Check sheet for the drawn part. Datum: minimum x, y, z corner. Units: mm. A direction names the side the tool comes from. Give positions to 0.01 mm unless a question says otherwise; leave off trailing zeros. Write each loop counter-clockwise with the first axis right and the second up, starting at its lowest first coordinate (ties: lowest second). Pieces come first, ordered by that corner, then holes. Notation, with made-up numbers: (22, 60.25) -> (66, 60.25) arc R24 ccw to (66, 86.25) -> close; hole circle Ø3 at (-30, -9). An arc over 180 degrees is marked (long way). Use CSV: the item, a comma, the result in double quotes. Start each with the question number.
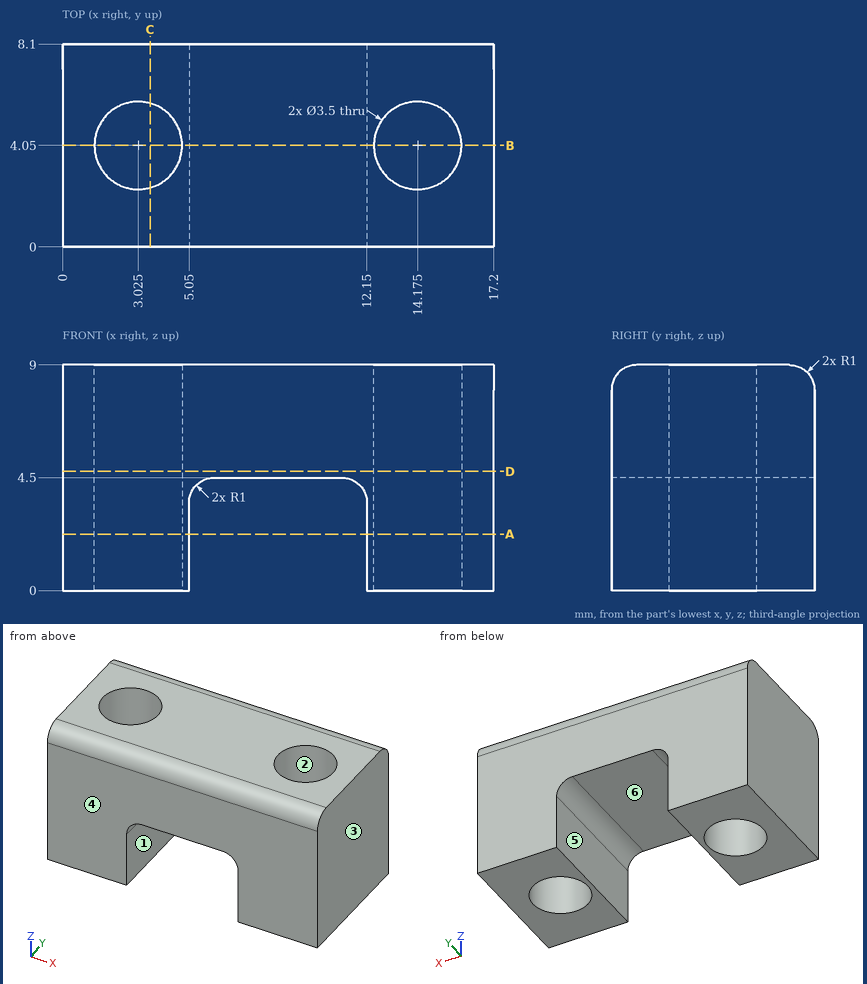
(1) Thickness scan on line 1 (X direction, y = 1.5, z = 1.5); line 2 (X direction, y = 5.5, z = 2.75); line 3 (X direction, y = 3.5, z = 0.75). Record the ranges inside material, lowest first. Write a range as from..to.
(2) Section check C-C on x = 3.5. Record the cut outline in (y, z), then the cut area to 3 significant figures.
(3) Draft check along X on the marked faces 3, 4, 5 and 6. Enter one of: released by +X, released by -X, zero draft, split by the parting line, or undercut.
(4) Set-up check for the marked faces 1 and 2: record each of +Z, -Z, +X, -X, +Y, -Y from which the full face is reachable in a straight line by a thin tool's end or side.
(5) Section check B-B on y = 4.05. Record the cut outline in (x, z) (3 decimals), then the cut area to 3 significant figures.
(6) Section check A-A on z = 2.25. Record the cut outline in (x, y) (3 decimals), then the cut area to 3 significant figures.
(7) Go/stop test with a flat-tipped pin: pin 1 (1.5 mm diameter, centred on x = 8.5, y = 5, fed in from -Z). Record where the tip stops, or that it passes through.
(8) Section check D-D on z = 4.75. Record the cut outline in (x, y) (3 decimals), then the cut area to 3 significant figures.
Data:
1,line 1,"x = 0..5.05, 12.15..17.2"
1,line 2,"x = 0..2.05, 4..5.05, 12.15..13.2, 15.15..17.2"
1,line 3,"x = 0..1.36, 4.69..5.05, 12.15..12.51, 15.84..17.2"
2,outline,"(0, 0) -> (2.37, 0) -> (2.37, 9) -> (1, 9) arc R1 ccw to (0, 8) -> close; (5.73, 0) -> (8.1, 0) -> (8.1, 8) arc R1 ccw to (7.1, 9) -> (5.73, 9) -> close"
2,area,"42.2 mm2"
3,face 3,"released by +X"
3,face 4,"zero draft"
3,face 5,"undercut"
3,face 6,"undercut"
4,face 1,"-Z, +Y, -Y"
4,face 2,"+Z, -Z"
5,outline,"(0, 0) -> (1.275, 0) -> (1.275, 9) -> (0, 9) -> close; (4.775, 0) -> (5.05, 0) -> (5.05, 3.5) arc R1 cw to (6.05, 4.5) -> (11.15, 4.5) arc R1 cw to (12.15, 3.5) -> (12.15, 0) -> (12.425, 0) -> (12.425, 9) -> (4.775, 9) -> close; (15.925, 0) -> (17.2, 0) -> (17.2, 9) -> (15.925, 9) -> close"
5,area,"60.3 mm2"
6,outline,"(0, 0) -> (5.05, 0) -> (5.05, 8.1) -> (0, 8.1) -> close; (12.15, 0) -> (17.2, 0) -> (17.2, 8.1) -> (12.15, 8.1) -> close; hole circle Ø3.5 at (3.025, 4.05); hole circle Ø3.5 at (14.175, 4.05)"
6,area,"62.6 mm2"
7,pin 1,"stops at z = 4.5"
8,outline,"(0, 0) -> (17.2, 0) -> (17.2, 8.1) -> (0, 8.1) -> close; hole circle Ø3.5 at (3.025, 4.05); hole circle Ø3.5 at (14.175, 4.05)"
8,area,"120 mm2"
